from build123d import *

# Parameters (mm, degrees)
MAINBODYS_W        = 20
MAINBODYS_H        = 28
MAIN_BODY_DEPTH    = 15
MB_FILLET_R        = 1
SHELL_START        = -9
SHELL_MB_OUTLINE_W = 28
SHELL_MB_OUTLINE_H = 27
SHELL_MB_DEPTH     = 18
TOP_BORE_REACH     = 36.583
TOPBORES_R         = 4
BOTTOMBORES_R      = 4.5
BOTTOM_BORE_DEPTH  = 34.7194306
MB_INNER_FILLET_R  = 0.2


# Read off the part's stored shape, not the designer's step: SHELL MB
with BuildPart() as part:
    # MainBodyS → MAIN BODY (new, symmetric)
    with BuildSketch(Plane(origin=(0, 0, 0), x_dir=(1, 0, 0), z_dir=(0, 1, 0))):
        Rectangle(MAINBODYS_W, MAINBODYS_H)
    extrude(amount=MAIN_BODY_DEPTH, both=True)

    # MB FILLET
    mb_fillet_edges = [part.edges().sort_by_distance(p)[0] for p in [
        (-10, 0, -14),
        (10, 0, -14),
    ]]
    fillet(mb_fillet_edges, radius=MB_FILLET_R)

    # SHELL MB outline → SHELL MB (cut)
    with BuildSketch(Plane.YZ.offset(SHELL_START)):
        with Locations((0, 0.5)):
            Rectangle(SHELL_MB_OUTLINE_W, SHELL_MB_OUTLINE_H)
    extrude(amount=SHELL_MB_DEPTH, mode=Mode.SUBTRACT)

    # TopBoreS → TOP BORE (cut, up to next)
    with BuildSketch(Plane(origin=(0, 15, 0), x_dir=(1, 0, 0), z_dir=(0, 1, 0)), mode=Mode.PRIVATE) as top_bore_sk1:
        with Locations(Location((0, 2, 0), (0, 0, 270))):
            Circle(TOPBORES_R)
    top_bore_tool1 = extrude(top_bore_sk1.sketch, amount=-TOP_BORE_REACH, mode=Mode.PRIVATE) & part.part
    add(top_bore_tool1.solids().sort_by_distance((0, 15, -2))[0], mode=Mode.SUBTRACT)

    # BottomBoreS → BOTTOM BORE (cut, through all)
    with BuildSketch(Plane(origin=(0, -14, 0), x_dir=(1, 0, 0), z_dir=(0, 1, 0))):
        with Locations(Location((0, 2, 0), (0, 0, 270))):
            Circle(BOTTOMBORES_R)
    extrude(amount=-BOTTOM_BORE_DEPTH, mode=Mode.SUBTRACT)

    # MB INNER FILLET
    mb_inner_fillet_edges = [part.edges().sort_by_distance(p)[0] for p in [
        (9, 0, -13),
        (-9, 0, -13),
    ]]
    fillet(mb_inner_fillet_edges, radius=MB_INNER_FILLET_R)


solid = part.part
Read the model definition and answer for the solid it produces. Units are mm, in the model's axes. A direction names the side the tool comes from. Round coordinates to 2 decimals unless told otherwise and drop trailing zeros. Write each loop counter-clockwise with the first axis right and the second up, starting at its lowest first coordinate (ties: lowest second). Pieces come first, ordered by that corner, then holes. Notation, with made-up numbers: (0.5, 20.5) - (53.5, 20.5) arc R20 cw to (53.5, 50.5) - close; hole circle Ø5 at (64, -35). An arc over 180 degrees is marked (long way). Use a Markdown table: item, result.
(1) The part is cut by section C-C (y = -4.75). Write down the section's boundary in (x, z), then the cut area to 3 significant figures.
Reported:
| item | result |
|---|---|
| outline | (-10, -13) arc R1 ccw to (-9, -14) - (9, -14) arc R1 ccw to (10, -13) - (10, 14) - (9, 14) - (9, -12.8) arc R0.2 cw to (8.8, -13) - (-8.8, -13) arc R0.2 cw to (-9, -12.8) - (-9, 14) - (-10, 14) - close |
| area | 73.6 mm2 |
(2) Straight lines are drawn through the part: line 1 along X through (y, z) = (-10, 7); line 2 along X through (y, z) = (14.25, -2); line 3 along Y through (x, z) = (7.5, -2). For each, find the intervals that lie inside material, in ascending order. Write a range as [from, to].
Reported:
| item | result |
|---|---|
| line 1 | [-10, -9], [9, 10] |
| line 2 | [-10, -4], [4, 10] |
| line 3 | [-15, -14], [14, 15] |
(3) The part is cut by section A-A (z = -2). Write down the section's boundary in (x, y).
Reported:
| item | result |
|---|---|
| outline | (-10, -15) - (-4.5, -15) - (-4.5, -14) - (-9, -14) - (-9, 14) - (-4, 14) - (-4, 15) - (-10, 15) - close; (4, 14) - (9, 14) - (9, -14) - (4.5, -14) - (4.5, -15) - (10, -15) - (10, 15) - (4, 15) - close |
(4) The part is cut by section B-B (x = 0). Write down the section's boundary in (y, z), then the cut area to 3 significant figures.
Reported:
| item | result |
|---|---|
| outline | (-15, -14) - (15, -14) - (15, -6) - (14, -6) - (14, -13) - (-14, -13) - (-14, -6.5) - (-15, -6.5) - close; (-15, 2.5) - (-14, 2.5) - (-14, 14) - (-15, 14) - close; (14, 2) - (15, 2) - (15, 14) - (14, 14) - close |
| area | 67.0 mm2 |
(5) This flat-tipped pin is pushed along its axis until it touches: pin 1 Ø2 at (x, y) = (-1, -8.5) entering from +Z. Where does it stop, or does it pass through?
Reported:
| item | result |
|---|---|
| pin 1 | z = -13 |
(6) The mould has two halves that part along Y. Classify faces 1 (the flat face through (0, -15, 3)), 2 (the cylindrical face through (9.715, -0.21, -13.699)), 3 (the flat face through (-9, 0, 1)): released by +Y, released by -Y, zero draft, split by the parting line, or undercut.
Reported:
| item | result |
|---|---|
| face 1 | released by -Y |
| face 2 | zero draft |
| face 3 | undercut |
(7) Which of the six approach directions +Z, -Z, +X, -X, +Y, -Y give full straight-line access (tool end or side, diameter ignored) to faces 4 (the flat face through (0, 15, 3)), 5 (the cylindrical face through (1.352, -14.493, 2.292)), 6 (the flat face through (0, 14, 3))?
Reported:
| item | result |
|---|---|
| face 4 | +Z, -Z, +X, -X, +Y |
| face 5 | -Y |
| face 6 | +Z |
(8) The part is cut by section D-D (z = 4). Write down the section's boundary in (x, y).
Reported:
| item | result |
|---|---|
| outline | (-10, -15) - (10, -15) - (10, 15) - (-10, 15) - close; hole (-9, -14) - (9, -14) - (9, 14) - (-9, 14) - close |
